Here's how the part is built. I have some questions about the finished solid (model axes, mm). A direction names the side the tool comes from. Round coordinates to 2 decimals unless told otherwise and drop trailing zeros. Order: outer loops, then holes, each group sorted by start corner. A loop starts at its lowest first (then second) coordinate and runs counter-clockwise, first axis right, second up. Notation, with made-up numbers: (-34.75, 32) - (-5.75, 32) arc R13 cw to (-5.75, 56) - close; hole circle Ø11 at (-15.5, -29). An arc over 180 degrees is marked (long way). One line per item, written item: value.
from build123d import *

# Parameters (mm, degrees)
F1_DEPTH = 10
F3_DEPTH = 10
F4_R     = 3
F5_DEPTH = 15


with BuildPart() as f1:
    # F0 (on Top) → F1 (new body)
    with BuildSketch(Plane.XY):
        with BuildLine():
            Line((5, 5.5), (-5, 5.5))
            ThreePointArc((-5, 5.5), (-7.12132, 4.62132), (-8, 2.5))
            Line((-8, 2.5), (-8, -2.5))
            ThreePointArc((-8, -2.5), (-7.12132, -4.62132), (-5, -5.5))
            Line((-5, -5.5), (5, -5.5))
            ThreePointArc((5, -5.5), (7.12132, -4.62132), (8, -2.5))
            Line((8, -2.5), (8, 2.5))
            ThreePointArc((8, 2.5), (7.12132, 4.62132), (5, 5.5))
        make_face()
    extrude(amount=F1_DEPTH)

    # F2 (on face) → F3 (join)
    with BuildSketch(Plane.XY.offset(10)):
        with BuildLine():
            Line((4.4, 4.9), (-4.4, 4.9))
            ThreePointArc((-4.4, 4.9), (-6.52132, 4.02132), (-7.4, 1.9))
            Line((-7.4, 1.9), (-7.4, -1.9))
            ThreePointArc((-7.4, -1.9), (-6.52132, -4.02132), (-4.4, -4.9))
            Line((-4.4, -4.9), (4.4, -4.9))
            ThreePointArc((4.4, -4.9), (6.52132, -4.02132), (7.4, -1.9))
            Line((7.4, -1.9), (7.4, 1.9))
            ThreePointArc((7.4, 1.9), (6.52132, 4.02132), (4.4, 4.9))
        make_face()
    extrude(amount=F3_DEPTH)

    # F4 (on face) → F5 (join)
    with BuildSketch(Plane(origin=(0, 0, 0), x_dir=(1, 0, 0), z_dir=(0, 0, -1))):
        Circle(F4_R)
    extrude(amount=F5_DEPTH)


solid = f1.part
Q1. If we section it at D-D, the plane z = -11: Please give me the cut outline in (x, y).
Results list:
outline: circle Ø6 at (0, 0)
Q2. If we section it at A-A, the plane x = 3.75: Please give me the cut outline in (y, z).
Results list:
outline: (-5.5, 0) - (5.5, 0) - (5.5, 10) - (4.9, 10) - (4.9, 20) - (-4.9, 20) - (-4.9, 10) - (-5.5, 10) - close
Q3. Will these pins go through, and if not, where does the flat tip stop? pin 1 (3 mm diameter, centred on x = -3, y = 1, fed in from -Z); pin 2 (2.5 mm diameter, centred on x = 1, z = 13, fed in from -Y); pin 3 (2.5 mm diameter, centred on x = -1, z = 17, fed in from +Y); pin 4 (4 mm diameter, centred on y = -0.5, z = 16, fed in from -X).
Results list:
pin 1: z = -15
pin 2: y = -4.9
pin 3: y = 4.9
pin 4: x = -7.4
Q4. If I drill on line 1 along Z through (x, y) = (-6.5, 0); line 2 along Z through (x, y) = (6.75, 4.25); line 3 along X through (y, z) = (-0.5, 16.5), over which ranges is the centre line in solid material (lowest first)?
Results list:
line 1: 0 to 20
line 2: 0 to 10
line 3: -7.4 to 7.4
Q5. Which directions (+Z, -Z, +X, -X, +Y, -Y) give clear straight access to the entire face, cutting with the end or side of a thin tool? Please do faces 1 (the flat face through (0, -4.9, 15)), 2 (the flat face through (-7.4, 0, 15)), 3 (the cylindrical face through (6.5, -4.04, 14.93)), 4 (the cylindrical face through (-3, 0, -7)).
Results list:
face 1: +Z, +X, -X, -Y
face 2: +Z, -X, +Y, -Y
face 3: +Z, +X, -Y
face 4: -Z
Q6. If we section it at B-B, the plane z = 9.5: Please give me the cut outline in (x, y).
Results list:
outline: (-8, -2.5) arc R3 ccw to (-5, -5.5) - (5, -5.5) arc R3 ccw to (8, -2.5) - (8, 2.5) arc R3 ccw to (5, 5.5) - (-5, 5.5) arc R3 ccw to (-8, 2.5) - close
Q7. If we section it at C-C, the plane x = 0: Please give me the cut outline in (y, z), then the cut area to 3 significant figures.
Results list:
outline: (-5.5, 0) - (-3, 0) - (-3, -15) - (3, -15) - (3, 0) - (5.5, 0) - (5.5, 10) - (4.9, 10) - (4.9, 20) - (-4.9, 20) - (-4.9, 10) - (-5.5, 10) - close
area: 298 mm²
